```python
from build123d import *

# Parameters (mm, degrees)
SM_BASE_FLANGE_1_DEPTH = 53
HOLE_WIZARD_M6_1_D     = 5
HOLE_WIZARD_M6_1_DEPTH = 3
HOLE_WIZARD_M6_1_TIP   = 1.502151548
HOLE_WIZARD_M6_2_D     = 5
HOLE_WIZARD_M6_2_DEPTH = 17
HOLE_WIZARD_M6_2_TIP   = 1.502151548
SKETCH_16_R            = 4.25
CUT_EXTRUDE_1_DEPTH    = 3
CHAMFER_1_SIZE         = 15
FILLET_1_R             = 10.68
FILLET_2_R             = 7.25


# Read off the part's stored shape, not the designer's step: 基体-法兰1
with BuildPart() as part:
    # 基体-法兰1 outline → 基体-法兰1 (new body)
    with BuildSketch(Plane.XY):
        with BuildLine():
            Line((15, 0), (15, 59.29))
            Line((15, 59.29), (12, 59.29))
            Line((12, 59.29), (12, 0))
            Line((12, 0), (0, 0))
            Line((0, 0), (0, -3))
            Line((0, -3), (12, -3))
            ThreePointArc((12, -3), (14.121320344, -2.121320344), (15, 0))
        make_face()
    extrude(amount=SM_BASE_FLANGE_1_DEPTH)

    # M6 螺纹孔1
    with Locations(Plane(origin=(15, 0, 0), x_dir=(0, 0, -1), z_dir=(1, 0, 0))):
        with Locations((-26.5, 54.35), (-48.42, 32.43), (-4.58, 32.43), (-36.5, 10), (-16.5, 10)):
            Hole(HOLE_WIZARD_M6_1_D / 2, depth=HOLE_WIZARD_M6_1_DEPTH)
            with Locations((0, 0, -(HOLE_WIZARD_M6_1_DEPTH + HOLE_WIZARD_M6_1_TIP / 2))):  # 118° drill point
                Cone(0, HOLE_WIZARD_M6_1_D / 2, HOLE_WIZARD_M6_1_TIP, mode=Mode.SUBTRACT)

    # M6 螺纹孔2
    with Locations(Plane(origin=(0, 0, 0), x_dir=(1, 0, 0), z_dir=(0, 1, 0))):
        with Locations((6, -6), (6, -47)):
            Hole(HOLE_WIZARD_M6_2_D / 2, depth=HOLE_WIZARD_M6_2_DEPTH)
            with Locations((0, 0, -(HOLE_WIZARD_M6_2_DEPTH + HOLE_WIZARD_M6_2_TIP / 2))):  # 118° drill point
                Cone(0, HOLE_WIZARD_M6_2_D / 2, HOLE_WIZARD_M6_2_TIP, mode=Mode.SUBTRACT)

    # 草图16 → 切除-拉伸1 (cut)
    with BuildSketch(Plane.ZY.offset(-12)):
        with Locations((26.5, 32)):
            Circle(SKETCH_16_R)
        with BuildLine():
            Line((44, 17.8), (44, 11))
            ThreePointArc((44, 11), (46.5, 8.5), (49, 11))
            Line((49, 11), (49, 17.8))
            ThreePointArc((49, 17.8), (46.5, 20.3), (44, 17.8))
        make_face()
        with BuildLine():
            Line((9, 17.8), (9, 11))
            ThreePointArc((9, 11), (6.5, 8.5), (4, 11))
            Line((4, 11), (4, 17.8))
            ThreePointArc((4, 17.8), (6.5, 20.3), (9, 17.8))
        make_face()
    extrude(amount=-CUT_EXTRUDE_1_DEPTH, mode=Mode.SUBTRACT)

    # 倒角1
    chamfer_1_edges = [part.edges().sort_by_distance(p)[0] for p in [
        (13.5, 59.29, 0),
        (13.5, 59.29, 53),
    ]]
    chamfer(chamfer_1_edges, length=CHAMFER_1_SIZE)

    # 圆角1
    fillet_1_edges = [part.edges().sort_by_distance(p)[0] for p in [
        (13.5, 59.29, 15),
        (13.5, 59.29, 38),
    ]]
    fillet(fillet_1_edges, radius=FILLET_1_R)

    # 圆角2
    fillet_2_edges = [part.edges().sort_by_distance(p)[0] for p in [
        (13.5, 44.29, 53),
        (13.5, 44.29, 0),
    ]]
    fillet(fillet_2_edges, radius=FILLET_2_R)


solid = part.part
```
Check sheet for the modelled part. Datum: model origin and axes. Units: mm. A direction names the side the tool comes from. Give positions to 0.01 mm unless a question says otherwise; leave off trailing zeros. Loops run counter-clockwise (first coordinate to the right, second up) from the corner with the lowest first, then second, coordinate; pieces in that order, holes last. Notation, with made-up numbers: M -6,66.5 L 46,66.5 A20 ccw 46,76.5 Z; hole C 28.5,8 d8. An arc over 180 degrees is marked long. Answer in a Markdown table with one row per item.
1) Thickness scan on line 1 (Z direction, x = 6, y = -0.9); line 2 (Y direction, x = 14.3, z = 26.5); line 3 (Y direction, x = 12.8, z = 26.5). Record the ranges inside material, lowest first.
Solutions:
| item | result |
|---|---|
| line 1 | z = 0 to 3.5, 8.5 to 44.5, 49.5 to 53 |
| line 2 | y = -1.93 to 27.75, 36.25 to 51.85, 56.85 to 59.29 |
| line 3 | y = -2.89 to 27.75, 36.25 to 51.85, 56.85 to 59.29 |
2) Cross-section at A-A (y = 54.35). Enter the section's corners in (x, z).
Solutions:
| item | result |
|---|---|
| outline | M 12,10.06 L 15,10.06 L 15,24 L 12,24 Z; M 12,29 L 15,29 L 15,42.94 L 12,42.94 Z |
3) Tool access check on faces 5 (the face through (13, 14, 44)), 6 (the face through (12, 23, 26)), 7 (the face through (13.479, 58.454, 15.283)). Record the directions out of +Z, -Z, +X, -X, +Y, -Y that give a thin tool (end or side, any length) a straight path to the whole face; none if there is none.
Solutions:
| item | result |
|---|---|
| face 5 | +X, -X |
| face 6 | +Z, -Z, -X, +Y |
| face 7 | -Z, +X, -X, +Y |
4) Cross-section at D-D (z = 36.5). Enter the section's corners in (x, y), plus the area to 3 significant figures.
Solutions:
| item | result |
|---|---|
| outline | M 0,-3 L 12,-3 A3 ccw 15,0 L 15,7.5 L 12,7.5 L 12,0 L 0,0 Z; M 12,12.5 L 15,12.5 L 15,58.88 L 12,58.88 Z |
| area | 205 mm^2 |
5) Cross-section at C-C (y = 33.5). Enter the section's corners in (x, z), plus the area to 3 significant figures.
Solutions:
| item | result |
|---|---|
| outline | M 12,0 L 15,0 L 15,2.32 L 12,2.32 Z; M 12,6.84 L 15,6.84 L 15,22.52 L 12,22.52 Z; M 12,30.48 L 15,30.48 L 15,46.16 L 12,46.16 Z; M 12,50.68 L 15,50.68 L 15,53 L 12,53 Z |
| area | 108 mm^2 |
6) Depth check by flat-ended pin: pin 1 (5 mm diameter, centred on y = 32, z = 26.5, fed in from -X) (3 decimals); pin 2 (8 mm diameter, centred on x = 10, z = 43.5, fed in from +Y) (3 decimals); pin 3 (5 mm diameter, centred on y = 10.5, z = 6, fed in from -X); pin 4 (3 mm diameter, centred on x = 3, z = 43.5, fed in from +Y). Enter the tip coordinate at first touch or a pass-through.
Solutions:
| item | result |
|---|---|
| pin 1 | passes through |
| pin 2 | stops at y = 57.115 |
| pin 3 | stops at x = 12 |
| pin 4 | stops at y = 0 |
7) Cross-section at B-B (z = 10.5). Enter the section's corners in (x, y), plus the area to 3 significant figures.
Solutions:
| item | result |
|---|---|
| outline | M 0,-3 L 12,-3 A3 ccw 15,0 L 15,54.79 L 12,54.79 L 12,0 L 0,0 Z |
| area | 207 mm^2 |
8) Mould release check, pull along X, two halves, no side actions. Record for faces 1 (the face through (0, -1, 26)), 2 (the face through (15, 23, 26)), 3 (the face through (6.54, -1.52, 49.44)), 4 (the face through (6, -3, 26)): released by +X, released by -X, zero draft, split by the parting line, or undercut.
Solutions:
| item | result |
|---|---|
| face 1 | released by -X |
| face 2 | released by +X |
| face 3 | undercut |
| face 4 | zero draft |
